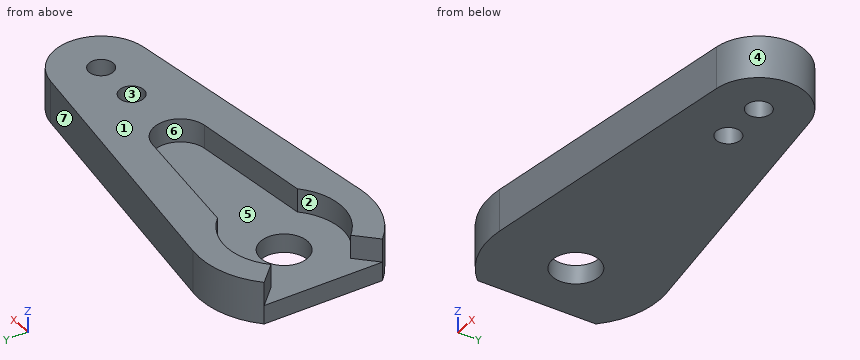
from build123d import *

# Parameters (mm, degrees)
MAIN_DEPTH            = 2.5
ESQUISSE2_R           = 2.5
ORIGINALBRACKET_DEPTH = 2
ESQUISSE3_R           = 1.3
FIXINGHOLE_DEPTH      = 5.5


with BuildPart() as part:
    # Esquisse1 → Main (new body)
    with BuildSketch(Plane.XY):
        with BuildLine():
            Line((-4.375785644, 4.25), (-6.426543071, 6.300757427))
            ThreePointArc((-6.426543071, 6.300757427), (-2.922982421, 8.512119229), (1.2, 8.919641248))
            Line((1.2, 8.919641248), (30.666666667, 4.955356249))
            ThreePointArc((30.666666667, 4.955356249), (35, 0), (30.666666667, -4.955356249))
            Line((30.666666667, -4.955356249), (1.2, -8.919641248))
            ThreePointArc((1.2, -8.919641248), (-2.922982421, -8.512119229), (-6.426543071, -6.300757427))
            Line((-6.426543071, -6.300757427), (-4.375785644, -4.25))
            ThreePointArc((-4.375785644, -4.25), (0, -6.1), (4.375785644, -4.25))
            Line((4.375785644, -4.25), (17.31559729, -2.78215714))
            ThreePointArc((17.31559729, -2.78215714), (19.8, 0), (17.31559729, 2.78215714))
            Line((17.31559729, 2.78215714), (4.375785644, 4.25))
            ThreePointArc((4.375785644, 4.25), (0, 6.1), (-4.375785644, 4.25))
        make_face()
    extrude(amount=MAIN_DEPTH)

    # Esquisse2 → OriginalBracket (add)
    with BuildSketch(Plane(origin=(0, 0, 0), x_dir=(-1, 0, 0), z_dir=(0, 0, -1))):
        with BuildLine():
            Line((-1.2, -8.919641248), (-30.666666667, -4.955356249))
            ThreePointArc((-30.666666667, -4.955356249), (-35, 0), (-30.666666667, 4.955356249))
            Line((-30.666666667, 4.955356249), (-1.2, 8.919641248))
            ThreePointArc((-1.2, 8.919641248), (2.922982421, 8.512119229), (6.426543071, 6.300757427))
            Line((6.426543071, 6.300757427), (6.426543071, -6.300757427))
            ThreePointArc((6.426543071, -6.300757427), (2.922982421, -8.512119229), (-1.2, -8.919641248))
        make_face()
        Circle(ESQUISSE2_R, mode=Mode.SUBTRACT)
    extrude(amount=ORIGINALBRACKET_DEPTH)

    # Esquisse3 → FixingHole (cut, through all)
    with BuildSketch(Plane.XY.offset(2.5)):
        with Locations((30, 0)):
            Circle(ESQUISSE3_R)
        with Locations((25, 0)):
            Circle(ESQUISSE3_R)
    extrude(amount=-FIXINGHOLE_DEPTH, mode=Mode.SUBTRACT)


solid = part.part
Work out the finished part from the listing and answer in its coordinate system (mm). Face numbers are marked on the shaded views. A direction names the side the tool comes from. Coordinates: 2 decimals unless noted, no trailing zeros. Write each loop counter-clockwise with the first axis right and the second up, starting at its lowest first coordinate (ties: lowest second). Pieces come first, ordered by that corner, then holes.
1. For the marked faces 5, 6 and 7, determine the directions among +Z, -Z, +X, -X, +Y, -Y from which every point of the face is accessible in a straight line to the end or side of a thin tool.
Results list:
face 5: +Z
face 6: +Z, -X
face 7: +Z, -Z, +X, +Y
2. Flat-ended cylindrical pins translate along their axes: pin 1 (1.5 mm diameter, centred on x = 7.5, y = -2.5, fed in from +Z); pin 2 (1.6 mm diameter, centred on x = 30, y = 0, fed in from -Z). Find the tip coordinate at first contact, or state that the pin passes through.
Results list:
pin 1: stops at z = 0
pin 2: passes through
3. Consider line 1 along X through (y, z) = (1, 0.45); line 2 along Y through (x, z) = (0, -0.8); line 3 along X through (y, z) = (-0.5, 1.95) (3 decimals). Determine where each line is inside the solid, lowest interval first.
Results list:
line 1: x = 19.62 to 24.17, 25.83 to 29.17, 30.83 to 34.9
line 2: y = -9 to -2.5, 2.5 to 9
line 3: x = 19.755 to 23.8, 26.2 to 28.8, 31.2 to 34.975
4. The part is cut by section B-B, the plane x = 0. Write down the section's boundary in (y, z), and give its area (3 significant figures).
Results list:
outline: (-9, -2) - (-2.5, -2) - (-2.5, 0) - (-6.1, 0) - (-6.1, 2.5) - (-9, 2.5) - close; (2.5, -2) - (9, -2) - (9, 2.5) - (6.1, 2.5) - (6.1, 0) - (2.5, 0) - close
area: 40.5 mm2
5. The part is cut by section D-D, the plane y = -2. Write down the section's boundary in (x, z).
Results list:
outline: (-6.43, -2) - (-1.5, -2) - (-1.5, 0) - (-6.43, 0) - close; (1.5, -2) - (34.58, -2) - (34.58, 2.5) - (18.96, 2.5) - (18.96, 0) - (1.5, 0) - close
6. The part is cut by section A-A, the plane y = 0. Write down the section's boundary in (x, z), and give its area (3 significant figures).
Results list:
outline: (-6.43, -2) - (-2.5, -2) - (-2.5, 0) - (-6.43, 0) - close; (2.5, -2) - (23.7, -2) - (23.7, 2.5) - (19.8, 2.5) - (19.8, 0) - (2.5, 0) - close; (26.3, -2) - (28.7, -2) - (28.7, 2.5) - (26.3, 2.5) - close; (31.3, -2) - (35, -2) - (35, 2.5) - (31.3, 2.5) - close
area: 87.5 mm2
7. For a pull along X with two mould halves and no side action, classify the marked faces 1, 2, 3 and 4 as +X half, -X half, draft (parallel to the pull), parting line (faces both ways), or undercut.
Results list:
face 1: draft
face 2: undercut
face 3: undercut
face 4: +X half
8. The part is cut by section C-C, the plane z = 1.15. Write down the section's boundary in (x, y).
Results list:
outline: (-6.43, -6.3) arc R9 ccw to (1.2, -8.92) - (30.67, -4.96) arc R5 ccw to (30.67, 4.96) - (1.2, 8.92) arc R9 ccw to (-6.43, 6.3) - (-4.38, 4.25) arc R6.1 cw to (4.38, 4.25) - (17.32, 2.78) arc R2.8 cw to (17.32, -2.78) - (4.38, -4.25) arc R6.1 cw to (-4.38, -4.25) - close; hole circle Ø2.6 at (25, 0); hole circle Ø2.6 at (30, 0)
